Can you work these out from the model? Positions are in its coordinate system, mm. Face numbers are marked on the shaded views. A direction names the side the tool comes from. Coordinates: 2 decimals unless noted, no trailing zeros. Order: outer loops, then holes, each group sorted by start corner. A loop starts at its lowest first (then second) coordinate and runs counter-clockwise, first axis right, second up. Notation, with made-up numbers: (-15.75, 15) - (-0.75, 15) arc R18 cw to (-0.75, 45) - close; hole circle Ø8 at (25, 6). An arc over 180 degrees is marked (long way). Return JSON: item names as keys, results as strings. Group by question number.
1) Imagine slicing it at D-D (y = -0.5). Write out the boundary of the cut face in (x, z) (3 decimals), and give its area (4 significant figures).
2) Imagine slicing it at A-A (x = -1.25). Write out the boundary of the cut face in (y, z), and give its area (3 significant figures).
3) Which directions (+Z, -Z, +X, -X, +Y, -Y) give clear straight access to the entire face, cutting with the end or side of a thin tool? Please do the marked faces 1 and 2.
4) Imagine slicing it at C-C (y = 2.25). Write out the boundary of the cut face in (x, z), and give its area (3 significant figures).
5) Imagine slicing it at B-B (z = 3). Write out the boundary of the cut face in (x, y), and give its area (3 significant figures).
```python
from build123d import *

# Parameters (mm, degrees)
SKETCH002_W     = 4.9
SKETCH002_H     = 0.1
SKETCH002_W_2   = 0.1
SKETCH002_H_2   = 6.1
SKETCH002_W_3   = 4.8
EXTRUDE_DEPTH   = 6.25
SKETCH003_W     = 1.25
SKETCH003_H     = 2.5
SKETCH003_W_2   = 2.25
SKETCH003_H_2   = 1.5
POCKET_DEPTH    = 5
FILLET_R        = 0.5
SKETCH005_W     = 6.5
SKETCH005_H     = 4
POCKET001_DEPTH = 5


with BuildPart() as part:
    # Sketch002 → Extrude (new body, symmetric)
    with BuildSketch(Plane.YZ):
        with Locations((0.65, 6.05)):
            Rectangle(SKETCH002_W, SKETCH002_H)
        with Locations((3.05, 2.95)):
            Rectangle(SKETCH002_W_2, SKETCH002_H_2)
        with Locations((0.6, -0.05)):
            Rectangle(SKETCH002_W_3, SKETCH002_H)
    extrude(amount=EXTRUDE_DEPTH, both=True)

    # Sketch003 (on Face9 of Extrude) → Pocket (cut)
    with BuildSketch(Plane.XY.offset(6.1)):
        with Locations((0, -0.55)):
            Rectangle(SKETCH003_W, SKETCH003_H)
        with Locations((3.25, -0.05)):
            Rectangle(SKETCH003_W_2, SKETCH003_H_2)
        with Locations((-3.25, -0.05)):
            Rectangle(SKETCH003_W_2, SKETCH003_H_2)
    extrude(amount=-POCKET_DEPTH, mode=Mode.SUBTRACT)

    # Fillet
    fillet_edges = [part.edges().sort_by_distance(p)[0] for p in [
        (0.625, -1.8, 6.05),
        (0.625, 0.7, 6.05),
        (-0.625, -1.8, 6.05),
        (-0.625, 0.7, 6.05),
        (6.25, -1.8, 6.05),
        (-6.25, -1.8, 6.05),
        (-6.25, -1.8, -0.05),
        (6.25, -1.8, -0.05),
    ]]
    fillet(fillet_edges, radius=FILLET_R)

    # Sketch005 (on Face4 of Fillet) → Pocket001 (cut)
    with BuildSketch(Plane.XZ.offset(-3)):
        with Locations((0, 3)):
            Rectangle(SKETCH005_W, SKETCH005_H)
    extrude(amount=-POCKET001_DEPTH, mode=Mode.SUBTRACT)


solid = part.part
```
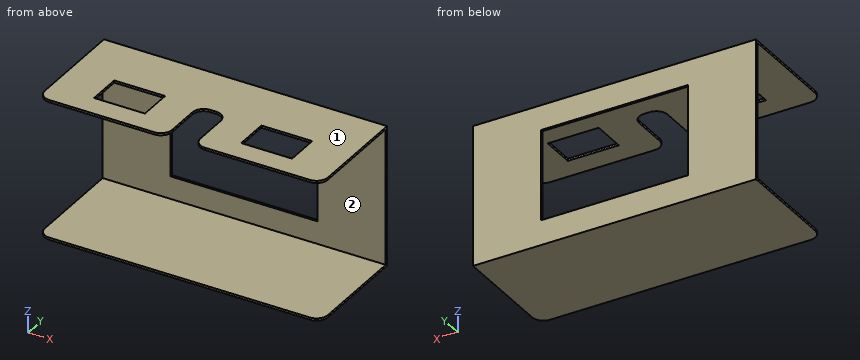
Calculated:
{
 "1": {"outline": "(-6.25, -0.1) - (6.25, -0.1) - (6.25, 0) - (-6.25, 0) - close; (-6.25, 6) - (-4.375, 6) - (-4.375, 6.1) - (-6.25, 6.1) - close; (-2.125, 6) - (-0.625, 6) - (-0.625, 6.1) - (-2.125, 6.1) - close; (0.625, 6) - (2.125, 6) - (2.125, 6.1) - (0.625, 6.1) - close; (4.375, 6) - (6.25, 6) - (6.25, 6.1) - (4.375, 6.1) - close", "area": "1.925 mm2"},
 "2": {"outline": "(-1.8, -0.1) - (3.1, -0.1) - (3.1, 1) - (3, 1) - (3, 0) - (-1.8, 0) - close; (-1.8, 6) - (3, 6) - (3, 5) - (3.1, 5) - (3.1, 6.1) - (-1.8, 6.1) - close", "area": "1.18 mm2"},
 "3": {"face 1": "+Z, +X, -X, +Y, -Y", "face 2": "+X, -X, -Y"},
 "4": {"outline": "(-6.25, -0.1) - (6.25, -0.1) - (6.25, 0) - (-6.25, 0) - close; (-6.25, 6) - (6.25, 6) - (6.25, 6.1) - (-6.25, 6.1) - close", "area": "2.50 mm2"},
 "5": {"outline": "(-6.25, 3) - (-3.25, 3) - (-3.25, 3.1) - (-6.25, 3.1) - close; (3.25, 3) - (6.25, 3) - (6.25, 3.1) - (3.25, 3.1) - close", "area": "0.600 mm2"}
}
